Source: CAD feature listing. Evaluate the final solid. Frame: model axes, mm. A direction names the side the tool comes from. Coordinates: 2 decimals unless noted, no trailing zeros. Loops run counter-clockwise (first coordinate to the right, second up) from the corner with the lowest first, then second, coordinate; pieces in that order, holes last.
from build123d import *

# Parameters (mm, degrees)
SKETCH1_W            = 65
SKETCH1_H            = 100
SKETCH1_R            = 10
BOSS_EXTRUDE1_DEPTH  = 14
SKETCH1_4_R          = 10
SKETCH1_4_R_2        = 5
BOSS_EXTRUDE3_DEPTH  = 1.5
SKETCH1_8_R          = 10
SKETCH1_8_R_2        = 5
BOSS_EXTRUDE6_DEPTH  = 14
SKETCH5_W            = 14
SKETCH5_H            = 40
SKETCH8_R            = 20
BOSS_EXTRUDE8_DEPTH  = 11.5
SKETCH11_R           = 15
BOSS_EXTRUDE10_DEPTH = 5
CUT_EXTRUDE1_REACH   = 118.045
SKETCH12_R           = 10
RIB1_START           = -6.5
RIB1_DEPTH           = 13
CUT_EXTRUDE2_DEPTH   = 15


# Read off the part's stored shape, not the designer's step: Rib1
with BuildPart() as part:
    # Sketch1 → Boss-Extrude1 (new body)
    with BuildSketch(Plane(origin=(0, 0, 0), x_dir=(1, 0, 0), z_dir=(0, 1, 0))):
        Rectangle(SKETCH1_W, SKETCH1_H)
        with Locations(Location((-18.5, 37, 0), (0, 0, 270))):
            Circle(SKETCH1_R, mode=Mode.SUBTRACT)
        with Locations(Location((18.5, -37, 0), (0, 0, 270))):
            Circle(SKETCH1_R, mode=Mode.SUBTRACT)
        with Locations(Location((-18.5, -37, 0), (0, 0, 270))):
            Circle(SKETCH1_R, mode=Mode.SUBTRACT)
        with Locations(Location((18.5, 37, 0), (0, 0, 270))):
            Circle(SKETCH1_R, mode=Mode.SUBTRACT)
    extrude(amount=-BOSS_EXTRUDE1_DEPTH)

    # Sketch1<4> → Boss-Extrude3 (add, symmetric)
    # profile 1 of 4: a face of its own
    with BuildSketch(Plane(origin=(0, 0, 0), x_dir=(1, 0, 0), z_dir=(0, 1, 0))):
        with Locations(Location((18.5, -37, 0), (0, 0, 270))):
            Circle(SKETCH1_4_R)
        with Locations(Location((18.5, -37, 0), (0, 0, 270))):
            Circle(SKETCH1_4_R_2, mode=Mode.SUBTRACT)
    # profile 2 of 4: a face of its own
    with BuildSketch(Plane(origin=(0, 0, 0), x_dir=(1, 0, 0), z_dir=(0, 1, 0))):
        with Locations(Location((-18.5, -37, 0), (0, 0, 270))):
            Circle(SKETCH1_4_R)
        with Locations(Location((-18.5, -37, 0), (0, 0, 270))):
            Circle(SKETCH1_4_R_2, mode=Mode.SUBTRACT)
    # profile 3 of 4: a face of its own
    with BuildSketch(Plane(origin=(0, 0, 0), x_dir=(1, 0, 0), z_dir=(0, 1, 0))):
        with Locations(Location((-18.5, 37, 0), (0, 0, 270))):
            Circle(SKETCH1_4_R)
        with Locations(Location((-18.5, 37, 0), (0, 0, 270))):
            Circle(SKETCH1_4_R_2, mode=Mode.SUBTRACT)
    # profile 4 of 4: a face of its own
    with BuildSketch(Plane(origin=(0, 0, 0), x_dir=(1, 0, 0), z_dir=(0, 1, 0))):
        with Locations(Location((18.5, 37, 0), (0, 0, 270))):
            Circle(SKETCH1_4_R)
        with Locations(Location((18.5, 37, 0), (0, 0, 270))):
            Circle(SKETCH1_4_R_2, mode=Mode.SUBTRACT)
    extrude(amount=BOSS_EXTRUDE3_DEPTH, both=True)

    # Sketch1<8> → Boss-Extrude6 (add)
    # profile 1 of 4: a face of its own
    with BuildSketch(Plane(origin=(0, 0, 0), x_dir=(1, 0, 0), z_dir=(0, 1, 0))):
        with Locations(Location((18.5, -37, 0), (0, 0, 270))):
            Circle(SKETCH1_8_R)
        with Locations(Location((18.5, -37, 0), (0, 0, 270))):
            Circle(SKETCH1_8_R_2, mode=Mode.SUBTRACT)
    # profile 2 of 4: a face of its own
    with BuildSketch(Plane(origin=(0, 0, 0), x_dir=(1, 0, 0), z_dir=(0, 1, 0))):
        with Locations(Location((-18.5, -37, 0), (0, 0, 270))):
            Circle(SKETCH1_8_R)
        with Locations(Location((-18.5, -37, 0), (0, 0, 270))):
            Circle(SKETCH1_8_R_2, mode=Mode.SUBTRACT)
    # profile 3 of 4: a face of its own
    with BuildSketch(Plane(origin=(0, 0, 0), x_dir=(1, 0, 0), z_dir=(0, 1, 0))):
        with Locations(Location((-18.5, 37, 0), (0, 0, 270))):
            Circle(SKETCH1_8_R)
        with Locations(Location((-18.5, 37, 0), (0, 0, 270))):
            Circle(SKETCH1_8_R_2, mode=Mode.SUBTRACT)
    # profile 4 of 4: a face of its own
    with BuildSketch(Plane(origin=(0, 0, 0), x_dir=(1, 0, 0), z_dir=(0, 1, 0))):
        with Locations(Location((18.5, 37, 0), (0, 0, 270))):
            Circle(SKETCH1_8_R)
        with Locations(Location((18.5, 37, 0), (0, 0, 270))):
            Circle(SKETCH1_8_R_2, mode=Mode.SUBTRACT)
    extrude(amount=-BOSS_EXTRUDE6_DEPTH)

    # Sweep1: sweep along a path in Sketch6
    with BuildLine(Plane.XY) as sweep1_path:
        Line((-32.5, 0), (-32.5, 12))
        ThreePointArc((-32.5, 12), (-36.893398282, 22.606601718), (-47.5, 27))
        Line((-47.5, 27), (-62.5, 27))
    # Sketch5 → Sweep1 (sweep)
    with BuildSketch(Plane(origin=(0, 0, 0), x_dir=(1, 0, 0), z_dir=(0, 1, 0))):
        with Locations((-25.5, 0)):
            Rectangle(SKETCH5_W, SKETCH5_H)
    sweep(path=sweep1_path.line)

    # Sketch8 → Boss-Extrude8 (add, symmetric)
    with BuildSketch(Plane(origin=(0, 34, 0), x_dir=(1, 0, 0), z_dir=(0, 1, 0))):
        with Locations(Location((-62.5, 0, 0), (0, 0, 270))):
            Circle(SKETCH8_R)
    extrude(amount=BOSS_EXTRUDE8_DEPTH, both=True)

    # Sketch11 → Boss-Extrude10 (add)
    with BuildSketch(Plane(origin=(0, 45.5, 0), x_dir=(1, 0, 0), z_dir=(0, 1, 0))):
        with Locations(Location((-62.5, 0, 0), (0, 0, 270))):
            Circle(SKETCH11_R)
    extrude(amount=BOSS_EXTRUDE10_DEPTH)

    # Sketch12 → Cut-Extrude1 (cut, up to next)
    with BuildSketch(Plane(origin=(0, 50.5, 0), x_dir=(1, 0, 0), z_dir=(0, 1, 0)), mode=Mode.PRIVATE) as cut_extrude1_sk1:
        with Locations(Location((-62.5, 0, 0), (0, 0, 270))):
            Circle(SKETCH12_R)
    cut_extrude1_tool1 = extrude(cut_extrude1_sk1.sketch, amount=-CUT_EXTRUDE1_REACH, mode=Mode.PRIVATE) & part.part
    add(cut_extrude1_tool1.solids().sort_by_distance((-62.5, 50.5, 0))[0], mode=Mode.SUBTRACT)

    # Rib1 outline → Rib1 (add)
    with BuildSketch(Plane.XY.offset(RIB1_START)):
        with BuildLine():
            Line((-50, 45.991191737), (-50, 41))
            Line((-50, 41), (-47.5, 41))
            ThreePointArc((-47.5, 41), (-26.993903346, 32.506096654), (-18.5, 12))
            Line((-18.5, 12), (-18.5, 0))
            Line((-18.5, 0), (32.5, 0))
            ThreePointArc((32.5, 0), (0.566198386, 31.925052284), (-42.5, 45.5))
            Line((-42.5, 45.5), (-48.981494165, 45.924487517))
            Line((-48.981494165, 45.924487517), (-50, 45.991191737))
        make_face()
    extrude(amount=RIB1_DEPTH)

    # Sketch14 → Cut-Extrude2 (cut, symmetric)
    with BuildSketch(Plane.XY):
        with BuildLine():
            Line((14.495933603, 6), (-8.980084126, 6))
            ThreePointArc((-8.980084126, 6), (-11.161205142, 6.940215761), (-11.975176588, 9.171525926))
            ThreePointArc((-11.975176588, 9.171525926), (-12.786554884, 18.744648632), (-16.243500658, 27.708606407))
            ThreePointArc((-16.243500658, 27.708606407), (-15.839776142, 31.196285594), (-12.402605555, 31.912356784))
            ThreePointArc((-12.402605555, 31.912356784), (3.209342465, 22.95318127), (16.699316747, 11.035952535))
            ThreePointArc((16.699316747, 11.035952535), (17.244374762, 7.797472995), (14.495933603, 6))
        make_face()
    extrude(amount=CUT_EXTRUDE2_DEPTH, both=True, mode=Mode.SUBTRACT)


solid = part.part
Q1. Section A-A, the plane z = -37. Return the cut outline in (x, y).
Q2. Contact query for flat-ended pins moving along their axis: pin 1 Ø4 at (x, y) = (-33.5, 33.5) entering from -Z; pin 2 Ø13 at (x, z) = (-9, 28.5) entering from +Y; pin 3 Ø2 at (x, y) = (-4, 31.5) entering from +Z. Output: stop coordinate, or through.
Q3. Section B-B, the plane z = 1.5. Return the cut outline in (x, y), plus the area to 3 significant figures.
Q4. Draft query along X for faces 1 (the cylindrical face through (-10.07, 0.74, 42.38)), 2 (the flat face through (-18.5, 6, 13)), 3 (the flat face through (0, -7, -50)). Return one class per face: +X half, -X half, draft (parallel to the pull), parting line (faces both ways), or undercut.
Q5. Section D-D, the plane y = 15.5. Return the cut outline in (x, z).
Q6. Access query for faces 4 (the flat face through (16, 1.5, -42)), 5 (the cylindrical face through (28.415, 0.74, 35.698)), 6 (the cylindrical face through (17.264, 7.842, 0.091)), 7 (the flat face through (-51, 41, -18)), 8 (the flat face through (16, 1.5, 32)). Directions: +Z, -Z, +X, -X, +Y, -Y. A direction counts if a zero-diameter tool reaches every point of the face in a straight line with its end or side. Return the directions, or none.
Q7. Line query: line 1 along Z through (x, y) = (18, -11); line 2 along X through (y, z) = (-0.95, 37); line 3 along X through (y, z) = (1.2, -37). Output: solid intervals per line, ascending.
Q8. Section C-C, the plane x = -20. Return the cut outline in (y, z).
Derived:
1. outline: (-32.5, -14) - (-23.5, -14) - (-23.5, 1.5) - (-28.5, 1.5) - (-28.5, 0) - (-32.5, 0) - close; (-13.5, -14) - (13.5, -14) - (13.5, 1.5) - (8.5, 1.5) - (8.5, 0) - (-8.5, 0) - (-8.5, 1.5) - (-13.5, 1.5) - close; (23.5, -14) - (32.5, -14) - (32.5, 0) - (28.5, 0) - (28.5, 1.5) - (23.5, 1.5) - close
2. pin 1: stops at z = -20
2. pin 2: stops at y = 1.5
2. pin 3: stops at z = 6.5
3. outline: (-82.44, 22.5) - (-72.39, 22.5) - (-72.39, 50.5) - (-77.42, 50.5) - (-77.42, 45.5) - (-82.44, 45.5) - close; (-52.61, 22.5) - (-42.56, 22.5) - (-42.56, 26.16) arc R15 cw to (-32.5, 12) - (-32.5, -14) - (32.5, -14) - (32.5, 0) arc R95 ccw to (-42.5, 45.5) - (-47.58, 45.83) - (-47.58, 50.5) - (-52.61, 50.5) - close; hole (-16.24, 27.71) arc R34 cw to (-11.98, 9.17) arc R3 ccw to (-8.98, 6) - (14.5, 6) arc R3 ccw to (16.7, 11.04) arc R89 ccw to (-12.4, 31.91) arc R3 ccw to start
3. area: 3,020 mm2
4. face 1: undercut
4. face 2: +X half
4. face 3: draft
5. outline: (-32.91, -20) - (-18.71, -20) - (-18.71, -6.5) - (-12.2, -6.5) - (-12.2, 6.5) - (-18.71, 6.5) - (-18.71, 20) - (-32.91, 20) - close; (12.27, -6.5) - (20.76, -6.5) - (20.76, 6.5) - (12.27, 6.5) - close
6. face 4: -Z, +X, -X, +Y
6. face 5: +Y
6. face 6: +Z, -Z
6. face 7: -Z, +X, +Y
6. face 8: +Z, +X, -X, +Y
7. line 1: z = -50 to -41.97, -32.03 to 32.03, 41.97 to 50
7. line 2: x = -32.5 to -23.5, -13.5 to 13.5, 23.5 to 32.5
7. line 3: x = -28.5 to -23.5, -13.5 to -8.5, 8.5 to 13.5, 23.5 to 28.5
8. outline: (-14, -50) - (0, -50) - (0, -46.89) - (1.5, -46.89) - (1.5, -41.77) - (-14, -41.77) - close; (-14, -32.23) - (1.5, -32.23) - (1.5, -27.11) - (0, -27.11) - (0, -20) - (21.21, -20) - (21.21, -6.5) - (41.26, -6.5) - (41.26, 6.5) - (21.21, 6.5) - (21.21, 20) - (0, 20) - (0, 27.11) - (1.5, 27.11) - (1.5, 32.23) - (-14, 32.23) - close; (-14, 41.77) - (1.5, 41.77) - (1.5, 46.89) - (0, 46.89) - (0, 50) - (-14, 50) - close
